```python
from build123d import *

# Parameters (mm, degrees)
CYLINDER017_R          = 2.5
CYLINDER017_DEPTH      = 25
CYLINDER016_R          = 5
CYLINDER016_DEPTH      = 5
CUT010_PLACEMENT_ANGLE = 90


with BuildPart() as rotor007:
    # Cylinder017 → Cylinder017 (new body)
    with BuildSketch(Plane(origin=(25, 25, 43), x_dir=(1, 0, 0), z_dir=(0, 0, 1))):
        Circle(CYLINDER017_R)
    extrude(amount=CYLINDER017_DEPTH)


with BuildPart() as e001:
    # Cylinder016 → Cylinder016 (new body)
    with BuildSketch(Plane(origin=(25, 25, 49), x_dir=(1, 0, 0), z_dir=(0, 0, 1))):
        Circle(CYLINDER016_R)
    extrude(amount=CYLINDER016_DEPTH)

    # Cut010: cut Rotor007
    add(rotor007.part, mode=Mode.SUBTRACT)


with BuildPart() as e001_1:
    # Cut010 placement: moved
    add(e001.part.moved(Location((11, -22.5, 55))).rotate(Axis((11, -22.5, 55), (0, 1, 0)), CUT010_PLACEMENT_ANGLE))


solid = e001_1.part
```
Can you work these out from the model? Positions are in its coordinate system, mm. Round coordinates to 2 decimals unless told otherwise and drop trailing zeros. Loops run counter-clockwise (first coordinate to the right, second up) from the corner with the lowest first, then second, coordinate; pieces in that order, holes last.
Item 1: If we mould it in two halves opening along Y, with no side actions, what happens to faces 1 (the cylindrical face through (62, 1, 32)), 2 (the flat face through (60, 5, 29)), 3 (the cylindrical face through (62.465, 2.72, 34.995))? For each: +Y half, -Y half, draft (parallel to the pull), parting line (faces both ways), or undercut.
Item 2: Will these pins go through, and if not, where does the flat tip stop? pin 1 Ø1 at (x, y) = (61, 0) entering from +Z; pin 2 Ø2 at (x, z) = (63, 28.5) entering from +Y; pin 3 Ø2 at (x, y) = (61.5, 0) entering from +Z.
Item 3: Suppose I cut it at D-D, the plane y = 5.5. Write out the boundary of the cut face in (x, z), then the cut area to 3 significant figures.
Item 4: Suppose I cut it at A-A, the plane y = 2.5. Write out the boundary of the cut face in (x, z).
Item 5: Please list where these lines run through material, in increasing order: L1, parallel to Y at x = 63.4, z = 30; L2, parallel to Z at x = 63, y = 4.75; L3, parallel to Z at x = 64.75, y = 4.5.
Item 6: Suppose I cut it at C-C, the plane x = 61.35. Write out the boundary of the cut face in (y, z).
Item 7: Suppose I cut it at B-B, the plane z = 30. Write out the boundary of the cut face in (x, y), then the cut area to 3 significant figures.
Reported:
1. face 1: undercut
1. face 2: draft
1. face 3: parting line
2. pin 1: stops at z = 34.58
2. pin 2: stops at y = 7.47
2. pin 3: stops at z = 34.77
3. outline: (60, 26) - (65, 26) - (65, 34) - (60, 34) - close
3. area: 40.0 mm2
4. outline: (60, 25) - (65, 25) - (65, 27.5) - (60, 27.5) - close; (60, 32.5) - (65, 32.5) - (65, 35) - (60, 35) - close
5. L1: y = -2.5 to 0, 5 to 7.5
5. L2: z = 25.53 to 28.91, 31.09 to 34.47
5. L3: z = 25.42 to 28.5, 31.5 to 34.58
6. outline: circle Ø10 at (2.5, 30); hole circle Ø5 at (2.5, 30)
7. outline: (60, -2.5) - (65, -2.5) - (65, 0) - (60, 0) - close; (60, 5) - (65, 5) - (65, 7.5) - (60, 7.5) - close
7. area: 25.0 mm2
